Could you check a few things on this model? Use its own coordinates, in mm. Face numbers are marked on the shaded views. A direction names the side the tool comes from. Coordinates: 2 decimals unless noted, no trailing zeros. Loops run counter-clockwise (first coordinate to the right, second up) from the corner with the lowest first, then second, coordinate; pieces in that order, holes last.
1) Imagine slicing it at D-D on y = 1.25. Please give me the cut outline in (x, z), plus the area to 3 significant figures.
2) Thinking about a two-plate mould opening in X: for the marked faces 4, 5 and 6, which applies, released by +X, released by -X, zero draft, split by the parting line, or undercut?
3) Imagine slicing it at C-C on y = -1.75. Please give me the cut outline in (x, z), plus the area to 3 significant figures.
4) For the marked faces 1, 2 and 3, which set-ups out of +Z, -Z, +X, -X, +Y, -Y let a thin tool reach every point of the face, with its end or its side?
5) If I drill on line 1 along X through (y, z) = (0, 2.8); line 2 along X through (y, z) = (0, 4.45), over which ranges is the centre line in solid material (lowest first)?
6) Will this pin go through, and if not, where does the flat tip stop? P1, Ø1.5, axis at x = 14, y = 2, coming from the +Z side.
7) Imagine slicing it at A-A on z = 0.45. Please give me the cut outline in (x, y), plus the area to 3 significant figures.
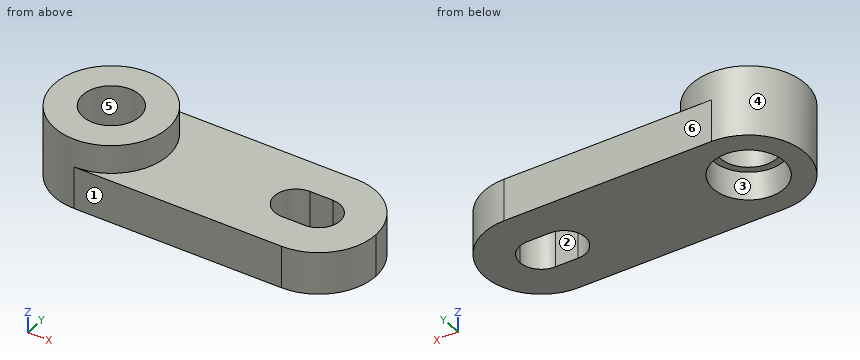
```python
from build123d import *

# Parameters (mm, degrees)
CROQUIS1_R              = 4
CROQUIS1_R_2            = 2
SALIENTE_EXTRUIR1_DEPTH = 3
CROQUIS2_R              = 4
CROQUIS2_R_2            = 2
SALIENTE_EXTRUIR2_DEPTH = 2
CROQUIS3_R              = 2.5
CORTAR_EXTRUIR1_DEPTH   = 2


with BuildPart() as part:
    # Croquis1 → Saliente-Extruir1 (new body)
    # profile 1 of 3: a face of its own
    with BuildSketch(Plane.XY):
        Circle(CROQUIS1_R)
        Circle(CROQUIS1_R_2, mode=Mode.SUBTRACT)
    # profile 2 of 3: a face of its own
    with BuildSketch(Plane.XY):
        with BuildLine():
            Line((14.5, 4), (0, 4))
            ThreePointArc((0, 4), (2.828427125, 2.828427125), (4, 0))
            ThreePointArc((4, 0), (2.828427125, -2.828427125), (0, -4))
            Line((0, -4), (14.5, -4))
            ThreePointArc((14.5, -4), (10.5, 0), (14.5, 4))
        make_face()
    # profile 3 of 3: a face of its own
    with BuildSketch(Plane.XY):
        with BuildLine():
            ThreePointArc((18.5, 0), (17.328427125, 2.828427125), (14.5, 4))
            ThreePointArc((14.5, 4), (10.5, 0), (14.5, -4))
            ThreePointArc((14.5, -4), (17.328427125, -2.828427125), (18.5, 0))
        make_face()
        with BuildLine():
            Line((14.5, -1.5), (12.9, -1.5))
            ThreePointArc((12.9, -1.5), (11.4, 0), (12.9, 1.5))
            Line((12.9, 1.5), (14.5, 1.5))
            ThreePointArc((14.5, 1.5), (15.560660172, 1.060660172), (16, 0))
            ThreePointArc((16, 0), (15.560660172, -1.060660172), (14.5, -1.5))
        make_face(mode=Mode.SUBTRACT)
    extrude(amount=SALIENTE_EXTRUIR1_DEPTH)

    # Croquis2 → Saliente-Extruir2 (add)
    with BuildSketch(Plane.XY.offset(3)):
        with Locations(Location((0, 0, 0), (0, 0, 270))):
            Circle(CROQUIS2_R)
        Circle(CROQUIS2_R_2, mode=Mode.SUBTRACT)
    extrude(amount=SALIENTE_EXTRUIR2_DEPTH)

    # Croquis3 → Cortar-Extruir1 (cut)
    with BuildSketch(Plane(origin=(0, 0, 0), x_dir=(-1, 0, 0), z_dir=(0, 0, -1))):
        Circle(CROQUIS3_R)
    extrude(amount=-CORTAR_EXTRUIR1_DEPTH, mode=Mode.SUBTRACT)


solid = part.part
```
Filled in:
1. outline: (-3.8, 0) - (-2.17, 0) - (-2.17, 2) - (-1.56, 2) - (-1.56, 5) - (-3.8, 5) - close; (1.56, 2) - (2.17, 2) - (2.17, 0) - (12.07, 0) - (12.07, 3) - (3.8, 3) - (3.8, 5) - (1.56, 5) - close; (15.33, 0) - (18.3, 0) - (18.3, 3) - (15.33, 3) - close
1. area: 53.7 mm2
2. face 4: split by the parting line
2. face 5: undercut
2. face 6: zero draft
3. outline: (-3.6, 0) - (-1.79, 0) - (-1.79, 2) - (-0.97, 2) - (-0.97, 5) - (-3.6, 5) - close; (0.97, 2) - (1.79, 2) - (1.79, 0) - (18.1, 0) - (18.1, 3) - (3.6, 3) - (3.6, 5) - (0.97, 5) - close
3. area: 66.5 mm2
4. face 1: +Z, -Z, +X, -X, -Y
4. face 2: +Z, -Z
4. face 3: -Z
5. line 1: x = -4 to -2, 2 to 11.4, 16 to 18.5
5. line 2: x = -4 to -2, 2 to 4
6. P1: stops at z = 3
7. outline: (0, -4) - (14.5, -4) arc R4 ccw to (14.5, 4) - (0, 4) arc R4 ccw to start; hole circle Ø5 at (0, 0); hole (12.9, -1.5) - (14.5, -1.5) arc R1.5 ccw to (14.5, 1.5) - (12.9, 1.5) arc R1.5 ccw to start
7. area: 135 mm2
